Geometry check sheet. Reference: drawing and pictorial views, mm from the part's lowest x, y, z. A direction names the side the tool comes from. Coordinates: 2 decimals unless noted, no trailing zeros. Write each loop counter-clockwise with the first axis right and the second up, starting at its lowest first coordinate (ties: lowest second). Pieces come first, ordered by that corner, then holes. Notation, with made-up numbers: (65.25, 76.25) - (82.25, 76.25) arc R16 ccw to (82.25, 87.25) - close; hole circle Ø3 at (48.5, 47.25). An arc over 180 degrees is marked (long way). Answer as CSV lines item,"result". Start each with the question number.
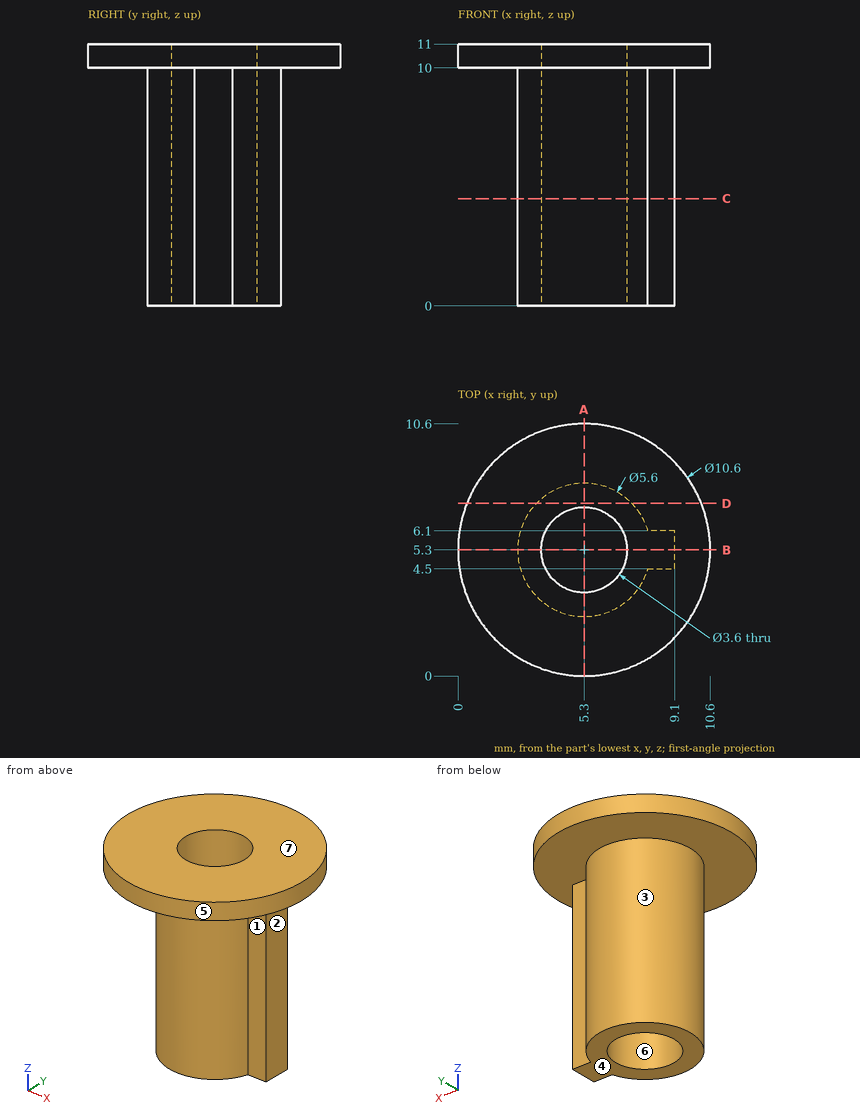
1. Draft check along X on the marked faces 5, 6 and 7. Enter one of: pulls with the +X half, pulls with the -X half, needs draft (parallel to the pull), parting line crosses it, or undercut.
2. Scan lines: line 1 along Y through (x, z) = (5.3, 4); line 2 along X through (y, z) = (3.75, 2.25); line 3 along Z through (x, y) = (5, 1.25). Record each from-to range of solid material in increasing order. Write a range as from..to.
3. Cross-section at A-A (x = 5.3). Record the cut outline in (y, z), and give its area (3 significant figures).
4. Depth check by flat-ended pin: P1, Ø5, axis at x = 3, z = 3, coming from the +Y side; P2, Ø0.6, axis at x = 8.5, z = 3, coming from the +Y side; P3, Ø1.3, axis at y = 5, z = 4, coming from the +X side; P4, Ø1.5, axis at y = 9, z = 6, coming from the +X side. Enter the tip coordinate at first touch or a pass-through.
5. Cross-section at B-B (y = 5.3). Record the cut outline in (x, z).
6. Cross-section at D-D (y = 7.25). Record the cut outline in (x, z).
7. Access from +Z, -Z, +X, -X, +Y, -Y to the whole of each face (thin tool, end or side, straight path). Record for the marked faces 1, 2, 3 and 4.
8. Cross-section at C-C (z = 4.5). Record the cut outline in (x, y), and give its area (3 significant figures).
Completed:
1,face 5,"parting line crosses it"
1,face 6,"undercut"
1,face 7,"needs draft"
2,line 1,"y = 2.5..3.5, 7.1..8.1"
2,line 2,"x = 2.97..4.38, 6.22..7.63"
2,line 3,"z = 10..11"
3,outline,"(0, 10) - (2.5, 10) - (2.5, 0) - (3.5, 0) - (3.5, 11) - (0, 11) - close; (7.1, 0) - (8.1, 0) - (8.1, 10) - (10.6, 10) - (10.6, 11) - (7.1, 11) - close"
3,area,"27.0 mm2"
4,P1,"stops at y = 8.1"
4,P2,"stops at y = 6.1"
4,P3,"stops at x = 9.1"
4,P4,"passes through"
5,outline,"(0, 10) - (2.5, 10) - (2.5, 0) - (3.5, 0) - (3.5, 11) - (0, 11) - close; (7.1, 0) - (9.1, 0) - (9.1, 10) - (10.6, 10) - (10.6, 11) - (7.1, 11) - close"
6,outline,"(0.37, 10) - (3.29, 10) - (3.29, 0) - (7.31, 0) - (7.31, 10) - (10.23, 10) - (10.23, 11) - (0.37, 11) - close"
7,face 1,"-Z, +X, -Y"
7,face 2,"-Z, +X, +Y, -Y"
7,face 3,"-Z"
7,face 4,"-Z, +X, -X, +Y, -Y"
8,outline,"(7.98, 4.5) - (9.1, 4.5) - (9.1, 6.1) - (7.98, 6.1) arc R2.8 ccw (long way) to start; hole circle Ø3.6 at (5.3, 5.3)"
8,area,"16.1 mm2"
